Here's how the part is built. I have some questions about the finished solid (model axes, mm). Face numbers are marked on the shaded views. A direction names the side the tool comes from. Round coordinates to 2 decimals unless told otherwise and drop trailing zeros. Loops run counter-clockwise (first coordinate to the right, second up) from the corner with the lowest first, then second, coordinate; pieces in that order, holes last. Notation, with made-up numbers: M 40,-0.5 L 64,-0.5 A15 cw 64,21.5 Z; hole C -33.75,82.25 d1. An arc over 180 degrees is marked long. One line per question, with ' | ' between items. Start each with the question number.
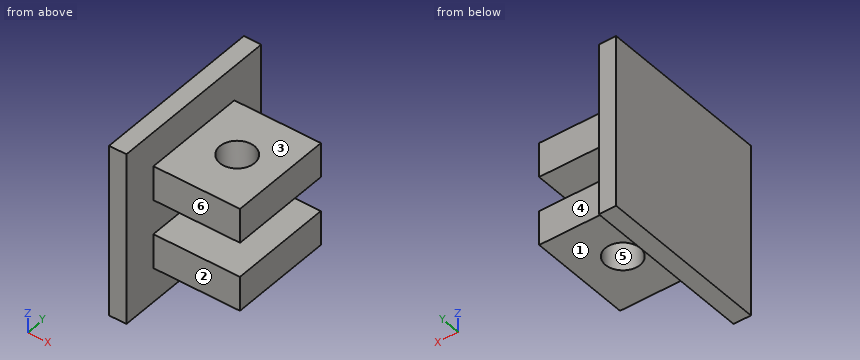
```python
from build123d import *

# Parameters (mm, degrees)
SKETCH5_W           = 100
SKETCH5_H           = 100
BOSS_EXTRUDE3_DEPTH = 10
SKETCH6_W           = 20
SKETCH6_H           = 60
BOSS_EXTRUDE4_DEPTH = 50
SKETCH7_R           = 10
CUT_EXTRUDE2_DEPTH  = 60


with BuildPart() as part:
    # Sketch5 → Boss-Extrude3 (new body)
    with BuildSketch(Plane(origin=(0, 0, 0), x_dir=(0, 0, -1), z_dir=(1, 0, 0))):
        Rectangle(SKETCH5_W, SKETCH5_H)
    extrude(amount=BOSS_EXTRUDE3_DEPTH)

    # Sketch6 → Boss-Extrude4 (add)
    with BuildSketch(Plane(origin=(10, 0, 0), x_dir=(0, 0, -1), z_dir=(1, 0, 0))):
        with Locations((-20, 0.076080003)):
            Rectangle(SKETCH6_W, SKETCH6_H)
        with Locations((20, 0)):
            Rectangle(SKETCH6_W, SKETCH6_H)
    extrude(amount=BOSS_EXTRUDE4_DEPTH)

    # Sketch7 → Cut-Extrude2 (cut)
    with BuildSketch(Plane.XY.offset(30)):
        with Locations((35, 0.076080003)):
            Circle(SKETCH7_R)
    extrude(amount=-CUT_EXTRUDE2_DEPTH, mode=Mode.SUBTRACT)


solid = part.part
```
1) Imagine slicing it at C-C (z = -21). Write out the boundary of the cut face in (x, y).
2) I'm going to push flat-ended pins straight in: pin 1 Ø5 at (x, z) = (25.5, 22.5) entering from +Y; pin 2 Ø15 at (x, y) = (40, 0.5) entering from +Z; pin 3 Ø2 at (x, y) = (26.5, 30) entering from -Z; pin 4 Ø18 at (x, y) = (35, 0.08) entering from -Z. Where does each tip first touch, or does it pass through?
3) Imagine slicing it at B-B (x = 56.5). Write out the boundary of the cut face in (y, z).
4) Imagine slicing it at A-A (x = 35). Write out the boundary of the cut face in (y, z).
5) Please list where these lines run through material, in increasing order: L1, parallel to Y at x = 35, z = -23; L2, parallel to Z at x = 12, y = 1; L3, parallel to Y at x = 35, z = 23. Write a range as from..to.
6) We'd pull the mould along Y, two halves only. Please class the marked faces 4, 5 and 6: pulls with the +Y half, pulls with the -Y half, needs draft (parallel to the pull), parting line crosses it, or undercut.
7) Imagine slicing it at D-D (y = 28). Write out the boundary of the cut face in (x, z), then the cut area to 3 significant figures.
8) For the marked faces 1, 2 and 3, which set-ups out of +Z, -Z, +X, -X, +Y, -Y let a thin tool reach every point of the face, with its end or its side?
Results are:
1) outline: M 0,-50 L 10,-50 L 10,-30 L 60,-30 L 60,30 L 10,30 L 10,50 L 0,50 Z; hole C 35,0.08 d20
2) pin 1: y = 30.08 | pin 2: z = 30 | pin 3: z = -30 | pin 4: through
3) outline: M -30,-30 L 30,-30 L 30,-10 L -30,-10 Z; M -29.92,10 L 30.08,10 L 30.08,30 L -29.92,30 Z
4) outline: M -30,-30 L -9.92,-30 L -9.92,-10 L -30,-10 Z; M -29.92,10 L -9.92,10 L -9.92,30 L -29.92,30 Z; M 10.08,-30 L 30,-30 L 30,-10 L 10.08,-10 Z; M 10.08,10 L 30.08,10 L 30.08,30 L 10.08,30 Z
5) L1: -30..-9.92, 10.08..30 | L2: -30..-10, 10..30 | L3: -29.92..-9.92, 10.08..30.08
6) face 4: pulls with the +Y half | face 5: undercut | face 6: pulls with the -Y half
7) outline: M 0,-50 L 10,-50 L 10,-30 L 60,-30 L 60,-10 L 10,-10 L 10,10 L 60,10 L 60,30 L 10,30 L 10,50 L 0,50 Z | area: 3,000 mm²
8) face 1: -Z, +X, +Y, -Y | face 2: +Z, -Z, +X, -Y | face 3: +Z, +X, +Y, -Y
